from build123d import *

# Parameters (mm, degrees)
BOSS_EXTRUDE1_DEPTH = 10
FILLET1_R           = 1
SKETCH2_W           = 21.86553483
SKETCH2_H           = 30.5
CUT_EXTRUDE1_DEPTH  = 5
MIRROR1_DEPTH       = 10
MIRROR1_2_OUTLINE_W = 21.86553483
MIRROR1_2_OUTLINE_H = 30.5
MIRROR1_2_DEPTH     = 5
SKETCH6_W           = 43.680332617
SKETCH6_H           = 16.249834628
CUT_EXTRUDE2_DEPTH  = 10


# Read off the part's stored shape, not the designer's step: Mirror1
with BuildPart() as part:
    # Sketch1 → Boss-Extrude1 (new body)
    with BuildSketch(Plane(origin=(0, 0, 0), x_dir=(1, 0, 0), z_dir=(0, 1, 0))):
        Polygon((-5, 57.097150921), (34.3, 57.097150921), (34.3, 55.097150921), (31.675, 55.097150921), (31.675, 52.597150921), (31.675, 2.599340873), (31.675, 0.099340873), (34.3, 0.099340873), (34.3, -4.5), (-5, -4.5), align=None)
        Polygon((-2.625, 45), (-2.625, 0), (-2.625, -2.5), (0, -2.5), (2.625, -2.5), (2.625, 0), (2.625, 45), (2.625, 47.5), (0, 47.5), (-2.625, 47.5), align=None, mode=Mode.SUBTRACT)
    extrude(amount=BOSS_EXTRUDE1_DEPTH)

    # Fillet1
    fillet1_edges = [part.edges().sort_by_distance(p)[0] for p in [
        (31.675, 5, -55.097150921),
        (31.675, 5, -0.099340873),
        (-2.625, 5, -47.5),
        (-2.625, 5, 2.5),
        (2.625, 5, 2.5),
        (2.625, 5, -47.5),
    ]]
    fillet(fillet1_edges, radius=FILLET1_R)

    # Sketch2 → Cut-Extrude1 (cut)
    with BuildSketch(Plane(origin=(0, 10, 0), x_dir=(1, 0, 0), z_dir=(0, 1, 0))):
        with Locations((20.742232585, 23.8519351)):
            Rectangle(SKETCH2_W, SKETCH2_H)
    extrude(amount=-CUT_EXTRUDE1_DEPTH, mode=Mode.SUBTRACT)

    # Mirror1 outline → Mirror1 (add)
    with BuildSketch(Plane(origin=(0, 0, 0), x_dir=(1, 0, 0), z_dir=(0, 1, 0))):
        with BuildLine():
            ThreePointArc((35.925, 55.097150921), (36.632106781, 54.804257702), (36.925, 54.097150921))
            Line((36.925, 54.097150921), (36.925, 39.1019351))
            Line((36.925, 39.1019351), (58.79053483, 39.1019351))
            Line((58.79053483, 39.1019351), (58.79053483, 8.6019351))
            Line((58.79053483, 8.6019351), (36.925, 8.6019351))
            Line((36.925, 8.6019351), (36.925, 1.099340873))
            ThreePointArc((36.925, 1.099340873), (36.632106781, 0.392234092), (35.925, 0.099340873))
            Line((35.925, 0.099340873), (34.3, 0.099340873))
            Line((34.3, 0.099340873), (34.3, -4.5))
            Line((34.3, -4.5), (73.6, -4.5))
            Line((73.6, -4.5), (73.6, 57.097150921))
            Line((73.6, 57.097150921), (34.3, 57.097150921))
            Line((34.3, 57.097150921), (34.3, 55.097150921))
            Line((34.3, 55.097150921), (35.925, 55.097150921))
        make_face()
        with BuildLine():
            Line((70.225, -2.5), (66.975, -2.5))
            ThreePointArc((66.975, -2.5), (66.267893219, -2.207106781), (65.975, -1.5))
            Line((65.975, -1.5), (65.975, 46.5))
            ThreePointArc((65.975, 46.5), (66.267893219, 47.207106781), (66.975, 47.5))
            Line((66.975, 47.5), (70.225, 47.5))
            ThreePointArc((70.225, 47.5), (70.932106781, 47.207106781), (71.225, 46.5))
            Line((71.225, 46.5), (71.225, -1.5))
            ThreePointArc((71.225, -1.5), (70.932106781, -2.207106781), (70.225, -2.5))
        make_face(mode=Mode.SUBTRACT)
    extrude(amount=MIRROR1_DEPTH)

    # Mirror1 2 outline → Mirror1 2 (add)
    with BuildSketch(Plane(origin=(0, 0, 0), x_dir=(1, 0, 0), z_dir=(0, 1, 0))):
        with Locations((47.857767415, 23.8519351)):
            Rectangle(MIRROR1_2_OUTLINE_W, MIRROR1_2_OUTLINE_H)
    extrude(amount=MIRROR1_2_DEPTH)

    # Sketch6 → Cut-Extrude2 (cut)
    with BuildSketch(Plane(origin=(0, 10, 0), x_dir=(1, 0, 0), z_dir=(0, 1, 0))):
        with Locations((61.699631479, -4.127511542)):
            Rectangle(SKETCH6_W, SKETCH6_H)
    extrude(amount=-CUT_EXTRUDE2_DEPTH, mode=Mode.SUBTRACT)


solid = part.part
Source: CAD feature listing. Evaluate the final solid. Frame: model axes, mm. A direction names the side the tool comes from. Coordinates: 2 decimals unless noted, no trailing zeros. Order: outer loops, then holes, each group sorted by start corner. A loop starts at its lowest first (then second) coordinate and runs counter-clockwise, first axis right, second up.
Item 1: Cut plane A-A (y = 2.25). Return loops of the section in (x, z) (3 decimals), plus the area to 3 significant figures.
Output values:
outline: (-5, -57.097) - (73.6, -57.097) - (73.6, -3.997) - (71.225, -3.997) - (71.225, -46.5) arc R1 cw to (70.225, -47.5) - (66.975, -47.5) arc R1 cw to (65.975, -46.5) - (65.975, -3.997) - (39.859, -3.997) - (39.859, 4.5) - (-5, 4.5) - close; hole (-2.625, -46.5) arc R1 ccw to (-1.625, -47.5) - (1.625, -47.5) arc R1 ccw to (2.625, -46.5) - (2.625, 1.5) arc R1 ccw to (1.625, 2.5) - (-1.625, 2.5) arc R1 ccw to (-2.625, 1.5) - close; hole (31.675, -54.097) arc R1 ccw to (32.675, -55.097) - (35.925, -55.097) arc R1 ccw to (36.925, -54.097) - (36.925, -1.099) arc R1 ccw to (35.925, -0.099) - (32.675, -0.099) arc R1 ccw to (31.675, -1.099) - close
area: 3,780 mm2
Item 2: Cut plane C-C (x = 42). Return loops of the section in (y, z), plus the area to 3 significant figures.
Output values:
outline: (0, -57.1) - (10, -57.1) - (10, -39.1) - (5, -39.1) - (5, -8.6) - (10, -8.6) - (10, -4) - (0, -4) - close
area: 378 mm2
Item 3: Cut plane D-D (z = -31). Return loops of the section in (x, y) (3 decimals).
Output values:
outline: (-5, 0) - (-2.625, 0) - (-2.625, 10) - (-5, 10) - close; (2.625, 0) - (31.675, 0) - (31.675, 5) - (9.809, 5) - (9.809, 10) - (2.625, 10) - close; (36.925, 0) - (65.975, 0) - (65.975, 10) - (58.791, 10) - (58.791, 5) - (36.925, 5) - close; (71.225, 0) - (73.6, 0) - (73.6, 10) - (71.225, 10) - close
Item 4: First-contact query: P1, Ø4, axis at x = 51, y = 3.5, coming from the +Z side; P2, Ø17.5, axis at x = 45.5, z = -29.5, coming from the +Y side. Flat tips, straight axial feed; report the tip coordinate or a pass-through.
Output values:
P1: stops at z = -4
P2: stops at y = 5
Item 5: Cut plane B-B (z = -52). Return loops of the section in (x, y) (3 decimals).
Output values:
outline: (-5, 0) - (31.675, 0) - (31.675, 10) - (-5, 10) - close; (36.925, 0) - (73.6, 0) - (73.6, 10) - (36.925, 10) - close
Item 6: Set-up query: faces 4 (the face through (65.975, 5, -25)), 5 (the face through (-5, 5, -26)), 6 (the face through (34, 5, -0.099)), 7 (the face through (48, 7, -8.602)), 8 (the face through (73.6, 5, -30)). Return all of +Z, -Z, +X, -X, +Y, -Y with unobstructed straight access to the full face (end or side cutting, diameter ignored); none if empty.
Output values:
face 4: +Z, +Y, -Y
face 5: +Z, -Z, -X, +Y, -Y
face 6: +Y, -Y
face 7: +Y
face 8: +Z, -Z, +X, +Y, -Y
Item 7: Material intervals for line 1 (X direction, y = 3.5, z = -17.5) (3 decimals); line 2 (X direction, y = 6, z = -10) (3 decimals); line 3 (Z direction, x = 0, y = 7.25), sorted ascending.
Output values:
line 1: x = -5 to -2.625, 2.625 to 31.675, 36.925 to 65.975, 71.225 to 73.6
line 2: x = -5 to -2.625, 2.625 to 9.809, 58.791 to 65.975, 71.225 to 73.6
line 3: z = -57.1 to -47.5, 2.5 to 4.5
Item 8: Pull-direction query (Z, two-part tool) for faces 1 (the face through (35, 5, -57.097)), 2 (the face through (25, 10, -40)), 3 (the face through (21, 5, -24)); classes: pulls with the +Z half, pulls with the -Z half, needs draft (parallel to the pull), parting line crosses it, or undercut.
Output values:
face 1: pulls with the -Z half
face 2: needs draft
face 3: undercut
